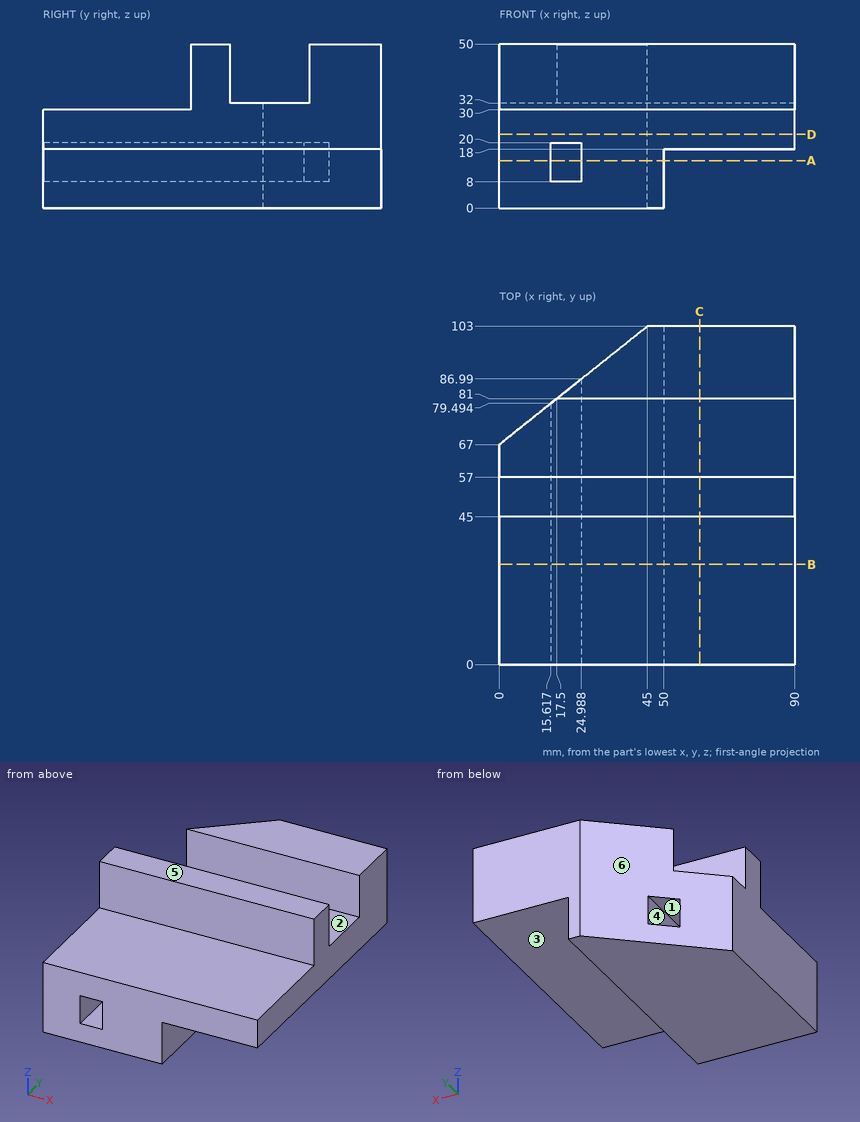
The drawing under review shows one solid part. Ordinate dimensions are in mm from its lowest x, y, z. A direction names the side the tool comes from. Coordinates: 2 decimals unless noted, no trailing zeros. Write each loop counter-clockwise with the first axis right and the second up, starting at its lowest first coordinate (ties: lowest second). Pieces come first, ordered by that corner, then holes. Notation, with made-up numbers: (12, 16) -> (50, 16) arc R16 ccw to (50, 21) -> close; hole circle Ø9 at (16.25, -36). An arc over 180 degrees is marked (long way). One line per item, written item: value. Start each with the question number.
Q1. Add section B-B, the plane y = 30.5. Give the boundary of the cut face in (x, z).
Q2. Add section C-C, the plane x = 61. Give the boundary of the cut face in (y, z), then the cut area to 3 significant figures.
Q3. For the marked faces 1, 2 and 3, list the 3-axis set-ups (+Z, -Z, +X, -X, +Y, -Y) from which the entire face can be reached by the end or side of a thin tool; tool diameter is ignored.
Q4. Clearance check with flat-ended pins moving along their axes: P1, Ø13.5, axis at x = 59.5, y = 28, coming from the +Z side; P2, Ø12, axis at x = 69.5, y = 31.5, coming from the -Z side; P3, Ø1.5, axis at x = 73.5, y = 73, coming from the +Z side; P4, Ø12, axis at x = 60.5, z = 10.5, coming from the -Y side. State where each tip first meets the part, or that it passes through.
Q5. Add section A-A, the plane z = 14.5. Give the boundary of the cut face in (x, y).
Q6. The part is to be moulded in two halves that separate along Z. For the marked faces 4, 5 and 6, say which applies: +Z half, -Z half, draft (parallel to the pull), parting line (faces both ways), or undercut.
Q7. To check wall thickness, follow probe 1 along Z at (x, y) = (19.5, 72.5); probe 2 along Z at (x, y) = (23, 8); probe 3 along Y at (x, z) = (86, 43). State the ranges of each line that lie inside material, in increasing order.
Q8. Add section D-D, the plane z = 22.5. Give the boundary of the cut face in (x, y), then the cut area to 3 significant figures.
Response:
1. outline: (0, 0) -> (50, 0) -> (50, 18) -> (90, 18) -> (90, 30) -> (0, 30) -> close; hole (15.62, 8) -> (24.99, 8) -> (24.99, 20) -> (15.62, 20) -> close
2. outline: (0, 18) -> (103, 18) -> (103, 50) -> (81, 50) -> (81, 32) -> (57, 32) -> (57, 50) -> (45, 50) -> (45, 30) -> (0, 30) -> close
2. area: 1,960 mm²
3. face 1: +Y, -Y
3. face 2: +Z, +X, -X
3. face 3: -Z, +X, +Y, -Y
4. P1: z = 30
4. P2: z = 18
4. P3: z = 32
4. P4: through
5. outline: (0, 0) -> (15.62, 0) -> (15.62, 79.49) -> (0, 67) -> close; (24.99, 0) -> (50, 0) -> (50, 103) -> (45, 103) -> (24.99, 86.99) -> close
6. face 4: undercut
6. face 5: +Z half
6. face 6: draft
7. probe 1: 0 to 8, 20 to 32
7. probe 2: 0 to 8, 20 to 30
7. probe 3: 45 to 57, 81 to 103
8. outline: (0, 0) -> (90, 0) -> (90, 103) -> (45, 103) -> (0, 67) -> close
8. area: 8,460 mm²
